Design review of the part shown in the three views and the two pictorial views. Dimensions are in mm from the part's minimum x, y and z. Round coordinates to 2 decimals unless told otherwise and drop trailing zeros. Loops run counter-clockwise (first coordinate to the right, second up) from the corner with the lowest first, then second, coordinate; pieces in that order, holes last. Notation, with made-up numbers: (0, -13.5) -> (23, -13.5) arc R32 ccw to (23, 13.5) -> close; hole circle Ø3 at (84, 25.25). An arc over 180 degrees is marked (long way). One line per question, with ' | ' between items. Start each with the question number.
1. For pin 1 Ø4 at (x, y) = (28.5, 4.5) entering from -Z; pin 2 Ø4 at (x, y) = (16, 6) entering from +Z, all flat-tipped, find the tip position at first contact; note any pin that passes through.
2. Consider section C-C (z = 0.35). Write out the cut boundary in (x, y), and give its area (3 significant figures).
3. Consider section B-B (y = 6). Write out the cut boundary in (x, z), and give its area (3 significant figures).
4. Wall thickness on line 1 along Y through (x, z) = (16, 1.15); line 2 along Y through (x, z) = (16.5, 0.7); line 3 along X through (y, z) = (6.25, 0.5): over which ranges is each line inside the solid? List them lowest first.
5. Consider section A-A (x = 16). Write out the cut boundary in (y, z).
6. Consider section D-D (z = 2). Write out the cut boundary in (x, y).
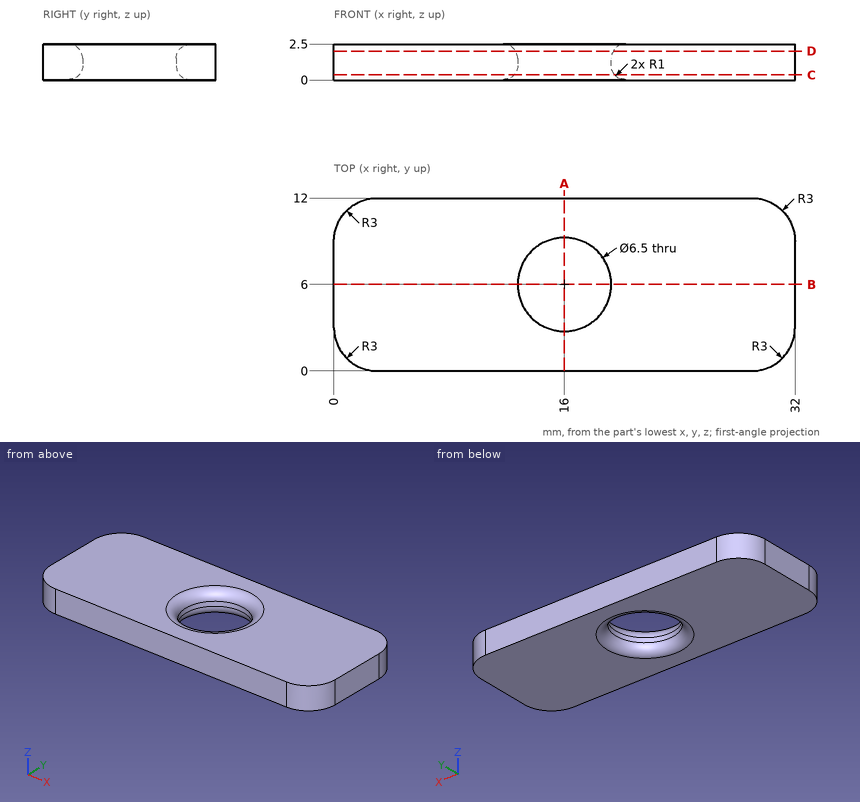
Answer block:
1) pin 1: stops at z = 0 | pin 2: passes through
2) outline: (0, 3) arc R3 ccw to (3, 0) -> (29, 0) arc R3 ccw to (32, 3) -> (32, 9) arc R3 ccw to (29, 12) -> (3, 12) arc R3 ccw to (0, 9) -> close; hole circle Ø6.98 at (16, 6) | area: 338 mm2
3) outline: (0, 0) -> (11.75, 0) arc R1 ccw to (12.75, 1) -> (12.75, 1.5) arc R1 ccw to (11.75, 2.5) -> (0, 2.5) -> close; (19.25, 1) arc R1 ccw to (20.25, 0) -> (32, 0) -> (32, 2.5) -> (20.25, 2.5) arc R1 ccw to (19.25, 1.5) -> close | area: 62.9 mm2
4) line 1: y = 0 to 2.75, 9.25 to 12 | line 2: y = 0 to 2.74, 9.26 to 12 | line 3: x = 0 to 12.63, 19.37 to 32
5) outline: (0, 0) -> (1.75, 0) arc R1 ccw to (2.75, 1) -> (2.75, 1.5) arc R1 ccw to (1.75, 2.5) -> (0, 2.5) -> close; (9.25, 1) arc R1 ccw to (10.25, 0) -> (12, 0) -> (12, 2.5) -> (10.25, 2.5) arc R1 ccw to (9.25, 1.5) -> close
6) outline: (0, 3) arc R3 ccw to (3, 0) -> (29, 0) arc R3 ccw to (32, 3) -> (32, 9) arc R3 ccw to (29, 12) -> (3, 12) arc R3 ccw to (0, 9) -> close; hole circle Ø6.77 at (16, 6)
